```python
from build123d import *

# Parameters (mm, degrees)
F2_T     = -1.27
F3_DEPTH = 1.27
F5_R     = 20.32
F6_DEPTH = 25.4
F7_W     = 1.905
F7_H     = 19.812
F8_DEPTH = 50.8


with BuildPart() as f1:
    # F0 (on Front) → F1 (revolve)
    with BuildSketch(Plane.XZ):
        Polygon((0, 63.5), (0, 0), (17.272, 0), (21.59, 63.5), align=None)
        Polygon((0, 66.04), (0, 63.5), (21.59, 63.5), (24.13, 63.5), (24.13, 66.04), align=None)
    revolve(axis=Axis((0, 0, 31.75), (0, 0, 1)))

    # F2
    f2_openings = [f1.faces().sort_by_distance(p)[0] for p in [
        (0, 0, 66.04),
    ]]
    offset(amount=F2_T, openings=f2_openings, kind=Kind.INTERSECTION)

    # F3 (add): a face of the model
    f3_faces = [f1.faces().sort_by_distance(p)[0] for p in [
        (-22.2134215593, 0, 64.77),
    ]]
    extrude(f3_faces, amount=F3_DEPTH)

    # F5 (on offset) → F6 (cut)
    with BuildSketch(Plane.XY.offset(63.5)):
        Circle(F5_R)
    extrude(amount=F6_DEPTH, mode=Mode.SUBTRACT)

    # F7 (on Top) → F8 (cut)
    with BuildSketch(Plane.XY):
        Polygon((0.9525, -27.178), (0.9525, -7.366), (0, -7.366), (-0.9525, -7.366), (-0.9525, -27.178), align=None)
        Polygon((5.2068558942, -5.3647039539), (3.6656785199, -6.4844348595), (15.3108799383, -22.5126795521), (16.8520573126, -21.3929486464), align=None)
        Polygon((7.4723698113, -1.2449737892), (6.883692437, -3.0567364527), (25.7260241378, -9.1789811453), (26.3147015121, -7.3672184818), align=None)
        Polygon((6.883692437, 3.4195935956), (7.4723698113, 1.6078309321), (26.3147015121, 7.7300756246), (25.7260241378, 9.5418382882), align=None)
        Polygon((3.6656785199, 6.8472920024), (5.2068558942, 5.7275610967), (16.8520573126, 21.7558057893), (15.3108799383, 22.8755366949), align=None)
        with Locations((0, 17.6348571429)):
            Rectangle(F7_W, F7_H)
        Polygon((-5.2068558942, 5.7275610967), (-3.6656785199, 6.8472920024), (-15.3108799383, 22.8755366949), (-16.8520573126, 21.7558057893), align=None)
        Polygon((-7.4723698113, 1.6078309321), (-6.883692437, 3.4195935956), (-25.7260241378, 9.5418382882), (-26.3147015121, 7.7300756246), align=None)
        Polygon((-6.883692437, -3.0567364527), (-7.4723698113, -1.2449737892), (-26.3147015121, -7.3672184818), (-25.7260241378, -9.1789811453), align=None)
        Polygon((-3.6656785199, -6.4844348595), (-5.2068558942, -5.3647039539), (-16.8520573126, -21.3929486464), (-15.3108799383, -22.5126795521), align=None)
    extrude(amount=F8_DEPTH, mode=Mode.SUBTRACT)

    # F9 (on Front) → F10 (revolve)
    with BuildSketch(Plane.XZ):
        Polygon((14.9047199998, 2.54), (14.732, 0), (17.272, 0), (17.44472, 2.54), align=None)
    revolve(axis=Axis((0, 0, 1.27), (0, 0, 1)))


solid = f1.part
```
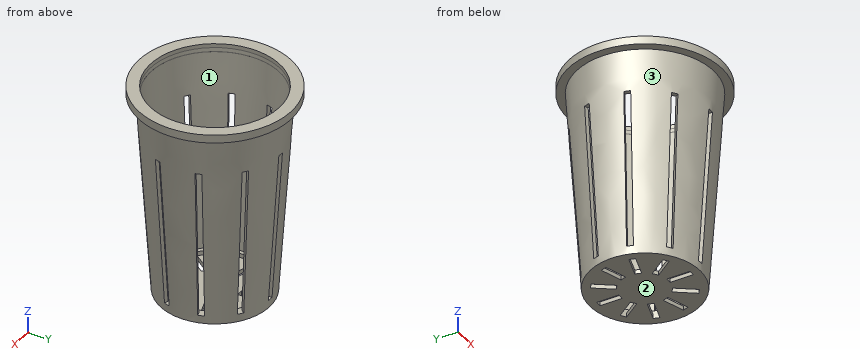
Can you work these out from the model? Positions are in its coordinate system, mm. Face numbers are marked on the shaded views. Round coordinates to 2 decimals unless told otherwise and drop trailing zeros. Loops run counter-clockwise (first coordinate to the right, second up) from the corner with the lowest first, then second, coordinate; pieces in that order, holes last. Notation, with made-up numbers: M 0.5,23.25 L 55.5,23.25 A23 cw 55.5,48.25 Z; hole C -39,36 d3. An arc over 180 degrees is marked long. Answer in a Markdown table with one row per item.
1. If we section it at B-B, the plane x = 0: Give the number of separate pieces and of enclosed holes in the cut face, plus the area to 3 significant figures.
Established:
| item | result |
|---|---|
| separate pieces | 5 |
| enclosed holes | 0 |
| area | 83.4 mm² |
2. Thinking about a two-plate mould opening in Y: for the marked faces 1, 2 and 3, which applies, pulls with the +Y half, pulls with the -Y half, needs draft (parallel to the pull), parting line crosses it, or undercut?
Established:
| item | result |
|---|---|
| face 1 | undercut |
| face 2 | needs draft |
| face 3 | parting line crosses it |
3. I'm going to push flat-ended pins straight in: pin 1 Ø3 at (x, y) = (1.5, 3) entering from -Z; pin 2 Ø1.4 at (x, z) = (0, 0.5) entering from -Y; pin 3 Ø10 at (x, z) = (13, 38) entering from -Y; pin 4 Ø1.4 at (y, z) = (-17.5, 21.5) entering from -X. Where does each tip first touch, or does it pass through?
Established:
| item | result |
|---|---|
| pin 1 | z = 0 |
| pin 2 | y = -17.35 |
| pin 3 | y = -18.2 |
| pin 4 | x = -8.29 |
4. Please list where these lines run through material, in increasing order: line 1 (Y direction, x = 0, z = 63.55); line 2 (Y direction, x = -16, z = 36); line 3 (X direction, y = -14, z = 32). Write a range as from..to.
Established:
| item | result |
|---|---|
| line 1 | -24.13..-20.32, 20.32..24.13 |
| line 2 | -11.53..-9.18, 9.18..11.53 |
| line 3 | -13.5..-11.59, 11.59..13.5 |
5. If we section it at C-C, the plane z = 61.5: Please give me the cut outline in (x, y), plus the area to 4 significant figures.
Established:
| item | result |
|---|---|
| outline | C 0,0 d42.91; hole C 0,0 d40.36 |
| area | 166.5 mm² |
